Autodesk Inventor part; units mm, degrees
ref_plane "YZ Plane" through (0, 0, 0) normal (1, 0, 0) x (0, 1, 0)
ref_plane "XZ Plane" through (0, 0, 0) normal (0, 1, 0) x (-1, 0, 0)
ref_plane "XY Plane" through (0, 0, 0) normal (0, 0, 1) x (1, 0, 0)
sketch "Sketch1" plane through (0, 0, 0) normal (0, 0, 1) x (1, 0, 0)
  line L0 (-61.8393, -52.0586) -> (-61.8393, 197.9414)
  line L1 (-11.8393, -52.0586) -> (-11.8393, 197.9414) construction
  line L2 (38.1607, -52.0586) -> (38.1607, 145.9423)
  line L3 (38.1607, -52.0586) -> (-61.8393, -52.0586)
  line L4 (43.1607, 183.0414) -> (38.1607, 183.0414)
  line L5 (43.1607, 172.9414) -> (43.1607, 183.0414)
  line L6 (38.1607, 172.9414) -> (43.1607, 172.9414)
  line L7 (43.1607, -16.9586) -> (38.1607, -16.9586)
  line L8 (43.1607, -27.0586) -> (43.1607, -16.9586)
  line L9 (38.1607, -27.0586) -> (43.1607, -27.0586)
  line L10 (-61.8393, 83.0414) -> (-61.8393, 72.9414)
  line L11 (-61.8393, 72.9414) -> (38.1607, 72.9414) construction
  line L12 (38.1607, 72.9414) -> (43.1607, 72.9414)
  line L13 (38.1607, 72.9414) -> (43.1607, 72.9414)
  line L14 (43.1607, 72.9414) -> (43.1607, 83.0414)
  line L15 (43.1607, 72.9414) -> (43.1607, 83.0414)
  line L16 (43.1607, 83.0414) -> (38.1607, 83.0414)
  line L17 (43.1607, 83.0414) -> (38.1607, 83.0414)
  line L18 (38.1607, 145.9423) -> (38.1607, 197.9414)
  line L19 (38.1607, 197.9414) -> (38.1607, 147.9414)
  line L20 (38.1607, 147.9414) -> (-61.8393, 147.9414) construction
  line L21 (-66.8393, -27.0586) -> (-66.8393, -16.9586)
  line L22 (-66.8393, -16.9586) -> (-61.8393, -16.9586)
  line L23 (-61.8393, -27.0586) -> (-66.8393, -27.0586)
  line L24 (-66.8393, 83.0414) -> (-61.8393, 83.0414)
  line L25 (-66.8393, 72.9414) -> (-66.8393, 83.0414)
  line L26 (-61.8393, 72.9414) -> (-66.8393, 72.9414)
  line L27 (-66.8393, 172.9414) -> (-66.8393, 183.0414)
  line L28 (-66.8393, 183.0414) -> (-61.8393, 183.0414)
  line L29 (-61.8393, 172.9414) -> (-66.8393, 172.9414)
  line L30 (-61.8393, 197.9414) -> (38.1607, 197.9414)
  line L31 (38.1607, 197.9414) -> (28.1607, 197.9414)
  line L32 (38.1607, 149.2033) -> (38.1607, 197.9414)
  line L33 (-61.8393, 197.9414) -> (-51.8393, 197.9414)
  line L34 (-61.8393, 149.2728) -> (-61.8393, 197.9414)
  line L35 (-61.8393, 147.9414) -> (38.1607, 147.9414) construction
  line L36 (28.1607, 145.2728) -> (28.1607, 139.2728)
  line L37 (17.1607, 145.2728) -> (17.1607, 139.2728)
  line L38 (-40.8393, 145.2728) -> (-40.8393, 139.2728)
  line L39 (-51.8393, 145.2728) -> (-51.8393, 139.2728)
  line L40 (17.1607, 145.2728) -> (-40.8393, 145.2728) construction
  line L41 (17.1607, 139.2728) -> (-40.8393, 139.2728) construction
  line L42 (28.1607, 139.2728) -> (17.1607, 139.2728)
  line L43 (28.1607, 145.2728) -> (17.1607, 145.2728)
  line L44 (-40.8393, 145.2728) -> (-51.8393, 145.2728)
  line L45 (-40.8393, 139.2728) -> (-51.8393, 139.2728)
  line L46 (-51.8393, 139.2728) -> (-61.8393, 139.2728) construction
  line L47 (-51.8393, 145.2728) -> (-61.8393, 145.2728) construction
  dimension "d8" = 10
  dimension "d9" = 11
extrude "Extrusion1" add sketch "Sketch1" along normal blind 5 contours L0 L30 L18 L2 L3 | L23 L21 L22 L0 | L2 L7 L8 L9 | L26 L25 L24 L0 | L2 L16 L14 L12 | L29 L27 L28 L0 | L18 L4 L5 L6 | L36 L42 L37 L43 | L38 L45 L39 L44
properties part number "Lifting Sections all back"
Read the model definition and answer for the solid it produces. Units are mm, in the model's axes. A direction names the side the tool comes from. Give positions to 0.01 mm unless a question says otherwise; leave off trailing zeros. Loops run counter-clockwise (first coordinate to the right, second up) from the corner with the lowest first, then second, coordinate; pieces in that order, holes last.
Item 1: Find the intervals of material crossed by line 1 along X through (y, z) = (-0.5, 0.5), in increasing order.
Item 2: Each of these flat-tipped pins is pushed along its axis until it touches: pin 1 Ø1.5 at (y, z) = (-39, 1.5) entering from +X; pin 2 Ø2.5 at (y, z) = (35.5, 2.5) entering from -X; pin 3 Ø2.5 at (x, z) = (41, 3) entering from -Y. Where does it stop, or does it pass through?
Item 3: The mould has two halves that part along Y. Classify faces 1 (the flat face through (43.161, 78, 2)), 2 (the flat face through (-11, -52.059, 2)), 3 (the flat face through (41, 72.941, 2)), 4 (the flat face through (41, -16.959, 2)): released by +Y, released by -Y, zero draft, split by the parting line, or undercut.
Item 4: The part is cut by section A-A (z = 1). Write down the section's boundary in (x, y).
Item 5: The part is cut by section B-B (y = 7). Write down the section's boundary in (x, z), and give its area (3 significant figures).
Item 6: For faces 5 (the flat face through (-64, 183.041, 2)), 6 (the flat face through (41, 183.041, 2)), 7 (the flat face through (-61.839, 27, 2)), 8 (the flat face through (41, 172.941, 2)), determine the directions among +Z, -Z, +X, -X, +Y, -Y from which every point of the face is accessible in a straight line to the end or side of a thin tool.
Taken from the geometry:
1. line 1: x = -61.84 to 38.16
2. pin 1: stops at x = 38.16
2. pin 2: stops at x = -61.84
2. pin 3: stops at y = -27.06
3. face 1: zero draft
3. face 2: released by -Y
3. face 3: undercut
3. face 4: undercut
4. outline: (-66.84, -27.06) - (-61.84, -27.06) - (-61.84, -52.06) - (38.16, -52.06) - (38.16, -27.06) - (43.16, -27.06) - (43.16, -16.96) - (38.16, -16.96) - (38.16, 72.94) - (43.16, 72.94) - (43.16, 83.04) - (38.16, 83.04) - (38.16, 172.94) - (43.16, 172.94) - (43.16, 183.04) - (38.16, 183.04) - (38.16, 197.94) - (-61.84, 197.94) - (-61.84, 183.04) - (-66.84, 183.04) - (-66.84, 172.94) - (-61.84, 172.94) - (-61.84, 83.04) - (-66.84, 83.04) - (-66.84, 72.94) - (-61.84, 72.94) - (-61.84, -16.96) - (-66.84, -16.96) - close
5. outline: (-61.84, 0) - (38.16, 0) - (38.16, 5) - (-61.84, 5) - close
5. area: 500 mm2
6. face 5: +Z, -Z, -X, +Y
6. face 6: +Z, -Z, +X, +Y
6. face 7: +Z, -Z, -X
6. face 8: +Z, -Z, +X
